Design review of the part built by this model. Coordinates are the model's own, in mm. A direction names the side the tool comes from. Coordinates: 2 decimals unless noted, no trailing zeros. Loops run counter-clockwise (first coordinate to the right, second up) from the corner with the lowest first, then second, coordinate; pieces in that order, holes last. Notation, with made-up numbers: (17.5, -7) -> (56.5, -7) arc R34 ccw to (56.5, 23) -> close; hole circle Ø10 at (-38, 78). An arc over 180 degrees is marked (long way). Answer as a JSON object with one key per item and string values.
```python
from build123d import *

# Parameters (mm, degrees)
SKETCH1_W           = 203.721686737
SKETCH1_H           = 149.733
BOSS_EXTRUDE1_DEPTH = 11.1125


with BuildPart() as part:
    # Sketch1 → Boss-Extrude1 (new body)
    with BuildSketch(Plane.XY):
        with Locations((-182.696343369, -43.420313263)):
            Rectangle(SKETCH1_W, SKETCH1_H)
        with BuildLine():
            Line((-242.774186737, -105.586813263), (-268.174186737, -105.586813263))
            ThreePointArc((-268.174186737, -105.586813263), (-271.857186737, -101.903813263), (-268.174186737, -98.220813263))
            Line((-268.174186737, -98.220813263), (-242.774186737, -98.220813263))
            ThreePointArc((-242.774186737, -98.220813263), (-239.091186737, -101.903813263), (-242.774186737, -105.586813263))
        make_face(mode=Mode.SUBTRACT)
        with BuildLine():
            Line((-242.774186737, -13.511813263), (-268.174186737, -13.511813263))
            ThreePointArc((-268.174186737, -13.511813263), (-271.857186737, -9.828813263), (-268.174186737, -6.145813263))
            Line((-268.174186737, -6.145813263), (-242.774186737, -6.145813263))
            ThreePointArc((-242.774186737, -6.145813263), (-239.091186737, -9.828813263), (-242.774186737, -13.511813263))
        make_face(mode=Mode.SUBTRACT)
        with BuildLine():
            Line((-150.699186737, -13.511813263), (-176.099186737, -13.511813263))
            ThreePointArc((-176.099186737, -13.511813263), (-179.782186737, -9.828813263), (-176.099186737, -6.145813263))
            Line((-176.099186737, -6.145813263), (-150.699186737, -6.145813263))
            ThreePointArc((-150.699186737, -6.145813263), (-147.016186737, -9.828813263), (-150.699186737, -13.511813263))
        make_face(mode=Mode.SUBTRACT)
        with BuildLine():
            Line((-150.699186737, -105.586813263), (-176.099186737, -105.586813263))
            ThreePointArc((-176.099186737, -105.586813263), (-179.782186737, -101.903813263), (-176.099186737, -98.220813263))
            Line((-176.099186737, -98.220813263), (-150.699186737, -98.220813263))
            ThreePointArc((-150.699186737, -98.220813263), (-147.016186737, -101.903813263), (-150.699186737, -105.586813263))
        make_face(mode=Mode.SUBTRACT)
        with BuildLine():
            Line((-196.736686737, -66.610669433), (-252.452295744, -66.610669433))
            ThreePointArc((-252.452295744, -66.610669433), (-263.196651914, -55.866313263), (-252.452295744, -45.121957093))
            Line((-252.452295744, -45.121957093), (-196.736686737, -45.121957093))
            ThreePointArc((-196.736686737, -45.121957093), (-185.992330568, -55.866313263), (-196.736686737, -66.610669433))
        make_face(mode=Mode.SUBTRACT)
    extrude(amount=BOSS_EXTRUDE1_DEPTH)


solid = part.part
```
1) For faces 4 (the cylindrical face through (-179.78, -9.91, 5.48)), 5 (the flat face through (-184, -118.287, 5)), list the 3-axis set-ups (+Z, -Z, +X, -X, +Y, -Y) from which the entire face can be reached by the end or side of a thin tool; tool diameter is ignored.
Completed:
{"face 4": "+Z, -Z", "face 5": "+Z, -Z, +X, -X, -Y"}
2) Add section B-B, the plane x = -166.5. Give the boundary of the cut face in (y, z).
Completed:
{"outline": "(-118.29, 0) -> (-105.59, 0) -> (-105.59, 11.11) -> (-118.29, 11.11) -> close; (-98.22, 0) -> (-13.51, 0) -> (-13.51, 11.11) -> (-98.22, 11.11) -> close; (-6.15, 0) -> (31.45, 0) -> (31.45, 11.11) -> (-6.15, 11.11) -> close"}
3) Add section A-A, the plane x = -211.5. Give the boundary of the cut face in (y, z), and give its area (3 significant figures).
Completed:
{"outline": "(-118.29, 0) -> (-66.61, 0) -> (-66.61, 11.11) -> (-118.29, 11.11) -> close; (-45.12, 0) -> (31.45, 0) -> (31.45, 11.11) -> (-45.12, 11.11) -> close", "area": "1,430 mm²"}
4) Wall thickness on probe 1 along Y at (x, z) = (-161, 10.75); probe 2 along Y at (x, z) = (-198, 1.5); probe 3 along Y at (x, z) = (-149.5, 10): over which ranges is each line inside the solid? List them lowest first.
Completed:
{"probe 1": "-118.29 to -105.59, -98.22 to -13.51, -6.15 to 31.45", "probe 2": "-118.29 to -66.61, -45.12 to 31.45", "probe 3": "-118.29 to -105.39, -98.42 to -13.31, -6.35 to 31.45"}
5) The part is to be moulded in two halves that separate along X. For faces 1 (the flat face through (-184, -42, 0)), 2 (the flat face through (-255, -13.512, 5)), 3 (the flat face through (-256, -6.146, 5)), say which applies: pulls with the +X half, pulls with the -X half, needs draft (parallel to the pull), parting line crosses it, or undercut.
Completed:
{"face 1": "needs draft", "face 2": "undercut", "face 3": "undercut"}
6) Add section C-C, the plane z = 1.75. Give the boundary of the cut face in (x, y).
Completed:
{"outline": "(-284.56, -118.29) -> (-80.84, -118.29) -> (-80.84, 31.45) -> (-284.56, 31.45) -> close; hole (-268.17, -105.59) -> (-242.77, -105.59) arc R3.68 ccw to (-242.77, -98.22) -> (-268.17, -98.22) arc R3.68 ccw to start; hole (-268.17, -13.51) -> (-242.77, -13.51) arc R3.68 ccw to (-242.77, -6.15) -> (-268.17, -6.15) arc R3.68 ccw to start; hole (-252.45, -66.61) -> (-196.74, -66.61) arc R10.74 ccw to (-196.74, -45.12) -> (-252.45, -45.12) arc R10.74 ccw to start; hole (-176.1, -105.59) -> (-150.7, -105.59) arc R3.68 ccw to (-150.7, -98.22) -> (-176.1, -98.22) arc R3.68 ccw to start; hole (-176.1, -13.51) -> (-150.7, -13.51) arc R3.68 ccw to (-150.7, -6.15) -> (-176.1, -6.15) arc R3.68 ccw to start"}
7) Add section D-D, the plane y = -51. Give the boundary of the cut face in (x, z), and give its area (3 significant figures).
Completed:
{"outline": "(-284.56, 0) -> (-262.03, 0) -> (-262.03, 11.11) -> (-284.56, 11.11) -> close; (-187.16, 0) -> (-80.84, 0) -> (-80.84, 11.11) -> (-187.16, 11.11) -> close", "area": "1,430 mm²"}
